Autodesk Inventor part; units mm, degrees
ref_plane "YZ Plane" through (0, 0, 0) normal (1, 0, 0) x (0, 1, 0)
ref_plane "XZ Plane" through (0, 0, 0) normal (0, 1, 0) x (-1, 0, 0)
ref_plane "XY Plane" through (0, 0, 0) normal (0, 0, 1) x (1, 0, 0)
sketch "Sketch94" plane through (0, 0, 0) normal (0, 1, 0) x (-1, 0, 0)
  line L0 (0, 0) -> (64, 0)
  line L1 (64, 0) -> (64, -49)
  line L2 (64, -49) -> (0, -49)
  line L3 (0, -49) -> (0, 0)
  dimension "d270" = 64
  dimension "d271" = 49
extrude "Extrusion51" add sketch "Sketch94" along normal blind 3
sketch "Sketch96" plane through (0, 0, 0) normal (0, -1, 0) x (1, 0, 0)
  line L0 (-64, 0) -> (0, 0)
  line L1 (0, 0) -> (-64, 0)
  line L2 (-64, 0) -> (-64, -3)
  line L3 (-64, -49) -> (-64, 0)
  line L4 (-64, -3) -> (0, -3)
  line L5 (0, -3) -> (0, 0)
  dimension "d274" = 3
extrude "Extrusion52" add sketch "Sketch96" along normal blind 31
sketch "Sketch97" plane through (0, 0, 0) normal (0, -1, 0) x (1, 0, 0)
  line L0 (0, -49) -> (-64, -49)
  line L1 (0, -49) -> (0, -46)
  line L2 (0, 0) -> (0, -49)
  line L3 (0, -46) -> (-64, -46)
  line L4 (-64, -49) -> (-64, 0)
  line L5 (-64, -49) -> (0, -49)
  dimension "d277" = 3
extrude "Extrusion53" add sketch "Sketch97" along normal blind 31
sketch "Sketch98" plane through (0, 3, 0) normal (0, 1, 0) x (1, 0, 0)
  line L0 (-64, 49) -> (0, 49)
  line L1 (0, 49) -> (-8, 49)
  line L2 (-8, 49) -> (-8, 42)
  line L3 (-8, 42) -> (0, 42)
  line L4 (0, 42) -> (0, 49)
  line L5 (-8, 42) -> (-28, 42)
  line L6 (-28, 42) -> (-28, 32)
  line L7 (-28, 32) -> (-8, 32)
  line L8 (-8, 32) -> (-8, 42)
  point P0 (0, 0)
  dimension "d280" = 8
  dimension "d281" = 7
  dimension "d282" = 20
  dimension "d283" = 10
extrude "Extrusion54" cut sketch "Sketch98" against normal blind 31 contours L8 L7 L6 L5
sketch "Sketch99" plane through (0, 3, 0) normal (0, 1, 0) x (1, 0, 0)
  line L0 (0, 0) -> (2, 0)
  line L1 (2, 0) -> (2, 49)
  line L2 (2, 49) -> (0, 49)
  line L3 (0, 49) -> (0, 0)
  dimension "d286" = 2
  dimension "d287" = 49
extrude "Extrusion55" add sketch "Sketch99" against normal blind 50
sketch "Sketch100" plane through (0, 0, 0) normal (0, -1, 0) x (1, 0, 0)
  line L0 (-64, -46) -> (-64, -3)
  line L1 (-64, -3) -> (0, -3)
  line L2 (-64, -46) -> (-61, -46)
  line L3 (-61, -46) -> (-61, -3)
  line L4 (-61, -3) -> (-64, -3)
  line L5 (-64, -3) -> (-64, -46)
  point P0 (0, 0)
  dimension "d290" = 3
extrude "Extrusion56" add sketch "Sketch100" along normal blind 13
sketch "Sketch101" plane through (2, 3, 0) normal (1, 0, 0) x (0, 0, -1)
  line L0 (0, -50) -> (49, -50)
  line L1 (0, -50) -> (24.5, -50)
  line L2 (24.5, -50) -> (24.5, -42)
  circle A0 centre (24.5, -42) radius 1.25
  point P0 (0, -3)
  dimension "d293" = 24.5
  dimension "d294" = 8
  dimension "d295" = 2.5
extrude "Extrusion57" cut sketch "Sketch101" against normal blind 13
properties part number "Back"
Check sheet for the modelled part. Datum: model origin and axes. Units: mm. A direction names the side the tool comes from. Give positions to 0.01 mm unless a question says otherwise; leave off trailing zeros. Loops run counter-clockwise (first coordinate to the right, second up) from the corner with the lowest first, then second, coordinate; pieces in that order, holes last. Notation, with made-up numbers: M -21.75,34 L 21.25,34 A21 cw 21.25,59 Z; hole C -22,28.5 d6. An arc over 180 degrees is marked long. Use a Markdown table: item, result. Add a question column.
Q1. Go/stop test with flat-tipped pins: pin 1 (12 mm diameter, centred on x = -23, z = -8.5, fed in from -Y); pin 2 (3 mm diameter, centred on y = -17, z = -17, fed in from -X); pin 3 (0.9 mm diameter, centred on x = -63, z = -17, fed in from -Y). Record where each tip stops, or that it passes through.
Q2. Sectioned sample at D-D, the plane x = -40. Record the cut outline in (y, z), then the cut area to 3 significant figures.
Q3. Sectioned sample at A-A, the plane z = -24.5. Record the cut outline in (x, y), then the cut area to 3 significant figures.
Q4. Sectioned sample at B-B, the plane y = -3.5. Record the cut outline in (x, z), then the cut area to 3 significant figures.
Q5. Scan lines: line 1 along Z through (x, y) = (-42.5, -30); line 2 along Z through (x, y) = (0.6, -39); line 3 along X through (y, z) = (-10.5, -26). Record each from-to range of solid material in increasing order. Write a range as [from, to].
Q6. Tool access check on faces 5 (the flat face through (-18, 2, -42)), 6 (the flat face through (-63, -13, -24)), 7 (the flat face through (-32, -31, -1)), 8 (the flat face through (-32, -15, -46)). Record the directions out of +Z, -Z, +X, -X, +Y, -Y that give a thin tool (end or side, any length) a straight path to the whole face; none if there is none.
Q7. Sectioned sample at C-C, the plane y = -39. Record the cut outline in (x, z).
Q8. Mould release check, pull along Z, two halves, no side actions. Record for faces 1 (the flat face through (-32, -31, -47)), 2 (the flat face through (-8, 2, -37)), 3 (the flat face through (-32, -15, -3)), 4 (the flat face through (-31, -11, 0)): pulls with the +Z half, pulls with the -Z half, needs draft (parallel to the pull), parting line crosses it, or undercut.
Verdict:
| question | item | result |
|---|---|---|
| 1 | pin 1 | y = -31 |
| 1 | pin 2 | x = 0 |
| 1 | pin 3 | y = -13 |
| 2 | outline | M -31,-49 L 3,-49 L 3,0 L -31,0 L -31,-3 L 0,-3 L 0,-46 L -31,-46 Z |
| 2 | area | 333 mm^2 |
| 3 | outline | M -64,-13 L -61,-13 L -61,0 L 0,0 L 0,-37.75 L 2,-37.75 L 2,3 L -64,3 Z; M 0,-47 L 2,-47 L 2,-40.25 L 0,-40.25 Z |
| 3 | area | 326 mm^2 |
| 4 | outline | M -64,-49 L 2,-49 L 2,0 L -64,0 Z; hole M -61,-46 L 0,-46 L 0,-3 L -61,-3 Z |
| 4 | area | 611 mm^2 |
| 5 | line 1 | [-49, -46], [-3, 0] |
| 5 | line 2 | [-49, -25.75], [-23.25, 0] |
| 5 | line 3 | [-64, -61], [0, 2] |
| 6 | face 5 | +Y, -Y |
| 6 | face 6 | -X, -Y |
| 6 | face 7 | +Z, -Z, -X, -Y |
| 6 | face 8 | -Y |
| 7 | outline | M 0,-49 L 2,-49 L 2,-25.75 L 0,-25.75 Z; M 0,-23.25 L 2,-23.25 L 2,0 L 0,0 Z |
| 8 | face 1 | needs draft |
| 8 | face 2 | undercut |
| 8 | face 3 | undercut |
| 8 | face 4 | pulls with the +Z half |
